The listing builds one solid part. Answer for the finished solid, in the listing's coordinates (mm). Face numbers are marked on the shaded views. A direction names the side the tool comes from. Coordinates: 2 decimals unless noted, no trailing zeros. Order: outer loops, then holes, each group sorted by start corner. A loop starts at its lowest first (then second) coordinate and runs counter-clockwise, first axis right, second up. Notation, with made-up numbers: (-14, 82) -> (42, 82) arc R20 cw to (42, 118) -> close; hole circle Ø1 at (-33.5, 32). An arc over 180 degrees is marked (long way). Answer in a Markdown table with one row per item.
```python
from build123d import *

# Parameters (mm, degrees)
F0_W     = 12
F0_H     = 12
F0_R     = 3.375
F1_DEPTH = 9.5
F2_DEPTH = 7.3
F3_DEPTH = 20


with BuildPart() as f1:
    # F0 (on Top) → F1 (new body)
    with BuildSketch(Plane.XY):
        Rectangle(F0_W, F0_H)
        Circle(F0_R, mode=Mode.SUBTRACT)
        Circle(F0_R)
        with BuildLine():
            ThreePointArc((-1.5, 2.5980762114), (1.5, 2.5980762114), (3, 0))
            ThreePointArc((3, 0), (1.5, -2.5980762114), (-1.5, -2.5980762114))
            ThreePointArc((-1.5, -2.5980762114), (-3, 0), (-1.5, 2.5980762114))
        make_face(mode=Mode.SUBTRACT)
        with BuildLine():
            ThreePointArc((-1.5, -2.5980762114), (1.5, -2.5980762114), (3, 0))
            ThreePointArc((3, 0), (1.5, 2.5980762114), (-1.5, 2.5980762114))
            Line((-1.5, 2.5980762114), (-1.5, -2.5980762114))
        make_face()
        with BuildLine():
            Line((-1.5, -2.5980762114), (-1.5, 2.5980762114))
            ThreePointArc((-1.5, 2.5980762114), (-3, 0), (-1.5, -2.5980762114))
        make_face()
    extrude(amount=-F1_DEPTH)

    # F0 (on Top) → F2 (join)
    with BuildSketch(Plane.XY):
        Circle(F0_R)
        with BuildLine():
            ThreePointArc((-1.5, 2.5980762114), (1.5, 2.5980762114), (3, 0))
            ThreePointArc((3, 0), (1.5, -2.5980762114), (-1.5, -2.5980762114))
            ThreePointArc((-1.5, -2.5980762114), (-3, 0), (-1.5, 2.5980762114))
        make_face(mode=Mode.SUBTRACT)
        with BuildLine():
            ThreePointArc((-1.5, -2.5980762114), (1.5, -2.5980762114), (3, 0))
            ThreePointArc((3, 0), (1.5, 2.5980762114), (-1.5, 2.5980762114))
            Line((-1.5, 2.5980762114), (-1.5, -2.5980762114))
        make_face()
        with BuildLine():
            Line((-1.5, -2.5980762114), (-1.5, 2.5980762114))
            ThreePointArc((-1.5, 2.5980762114), (-3, 0), (-1.5, -2.5980762114))
        make_face()
    extrude(amount=F2_DEPTH)

    # F0 (on Top) → F3 (join)
    with BuildSketch(Plane.XY):
        with BuildLine():
            ThreePointArc((-1.5, -2.5980762114), (1.5, -2.5980762114), (3, 0))
            ThreePointArc((3, 0), (1.5, 2.5980762114), (-1.5, 2.5980762114))
            Line((-1.5, 2.5980762114), (-1.5, -2.5980762114))
        make_face()
    extrude(amount=F3_DEPTH)


solid = f1.part
```
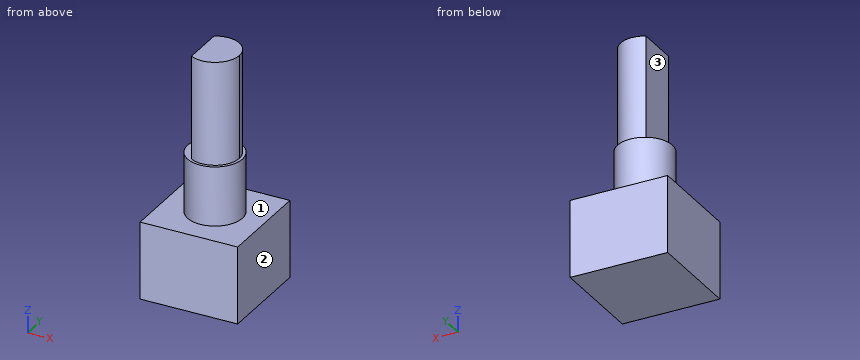
(1) Flat-ended cylindrical pins translate along their axes: pin 1 (1.5 mm diameter, centred on x = 3, z = 16, fed in from +Y); pin 2 (5.5 mm diameter, centred on y = -1, z = 16, fed in from -X); pin 3 (1.5 mm diameter, centred on x = 3.5, y = -2, fed in from +Z). Find the tip coordinate at first contact, or state that the pin passes through.
Check values:
| item | result |
|---|---|
| pin 1 | y = 1.98 |
| pin 2 | x = -1.5 |
| pin 3 | z = 7.3 |
(2) A cutting plane is placed at A-A, the plane x = 0. Determine the outline of the cut face in (y, z) (3 decimals), then the cut area to 3 significant figures.
Check values:
| item | result |
|---|---|
| outline | (-6, -9.5) -> (6, -9.5) -> (6, 0) -> (3.375, 0) -> (3.375, 7.3) -> (3, 7.3) -> (3, 20) -> (-3, 20) -> (-3, 7.3) -> (-3.375, 7.3) -> (-3.375, 0) -> (-6, 0) -> close |
| area | 239 mm² |
(3) A cutting plane is placed at C-C, the plane z = 2. Determine the outline of the cut face in (x, y) (3 decimals).
Check values:
| item | result |
|---|---|
| outline | circle Ø6.75 at (0, 0) |
(4) A cutting plane is placed at D-D, the plane x = 4.25. Determine the outline of the cut face in (y, z).
Check values:
| item | result |
|---|---|
| outline | (-6, -9.5) -> (6, -9.5) -> (6, 0) -> (-6, 0) -> close |
(5) A cutting plane is placed at B-B, the plane y = -1.75. Determine the outline of the cut face in (x, z), then the cut area to 3 significant figures.
Check values:
| item | result |
|---|---|
| outline | (-6, -9.5) -> (6, -9.5) -> (6, 0) -> (2.89, 0) -> (2.89, 7.3) -> (2.44, 7.3) -> (2.44, 20) -> (-1.5, 20) -> (-1.5, 7.3) -> (-2.89, 7.3) -> (-2.89, 0) -> (-6, 0) -> close |
| area | 206 mm² |
(6) Find the intervals of material crossed by line 1 along Z through (x, y) = (-3, -1.75); line 2 along Z through (x, y) = (-3.25, 0.75); line 3 along X through (y, z) = (-1.5, 8.25), in increasing order. Write a range as from..to.
Check values:
| item | result |
|---|---|
| line 1 | -9.5..0 |
| line 2 | -9.5..7.3 |
| line 3 | -1.5..2.6 |
(7) Which of the six approach directions +Z, -Z, +X, -X, +Y, -Y give full straight-line access (tool end or side, diameter ignored) to the marked faces 1, 2 and 3?
Check values:
| item | result |
|---|---|
| face 1 | +Z |
| face 2 | +Z, -Z, +X, +Y, -Y |
| face 3 | +Z, -X, +Y, -Y |
